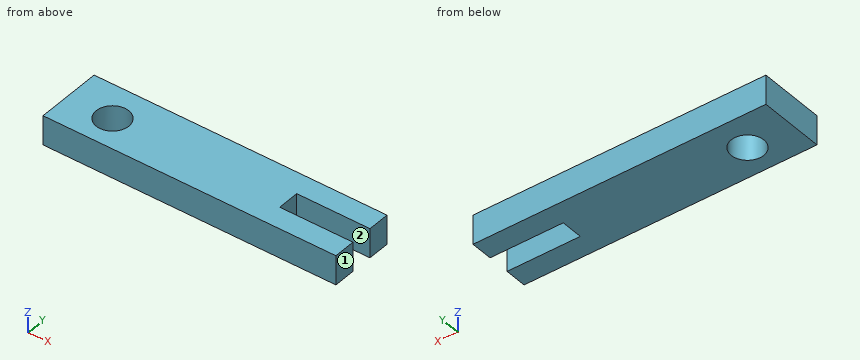
```python
from build123d import *

# Parameters (mm, degrees)
CROQUIS1_W              = 350
CROQUIS1_H              = 20
SALIENTE_EXTRUIR1_DEPTH = 45
CROQUIS2_R              = 11.125
CORTAR_EXTRUIR1_DEPTH   = 182.796589627
CROQUIS3_R              = 11.125
CORTAR_EXTRUIR2_DEPTH   = 182.796589627


with BuildPart() as part:
    # Croquis1 → Saliente-Extruir1 (new body)
    with BuildSketch(Plane(origin=(0, 0, 0), x_dir=(1, 0, 0), z_dir=(0, 1, 0))):
        Rectangle(CROQUIS1_W, CROQUIS1_H)
    extrude(amount=SALIENTE_EXTRUIR1_DEPTH)

    # Croquis2 → Cortar-Extruir1 (cut, through all)
    with BuildSketch(Plane(origin=(0, 0, -10), x_dir=(-1, 0, 0), z_dir=(0, 0, -1))):
        with Locations((-143.9, 21.1)):
            Circle(CROQUIS2_R)
    cortar_extruir1 = extrude(amount=-CORTAR_EXTRUIR1_DEPTH, mode=Mode.SUBTRACT)

    # Simetría1: Cortar-Extruir1 across plane
    add(cortar_extruir1.mirror(Plane(origin=(0, 0, 0), x_dir=(0, 0, 1), z_dir=(1, 0, 0))), mode=Mode.SUBTRACT)

    # Croquis3 → Cortar-Extruir2 (cut, through all)
    with BuildSketch(Plane.XY.offset(10)):
        Polygon((25, 15), (25, 0), (175, 0), (175, 45), (25, 45), (25, 30), (-25, 30), (-25, 15), align=None)
        with Locations((143.9, 21.1)):
            Circle(CROQUIS3_R, mode=Mode.SUBTRACT)
    extrude(amount=-CORTAR_EXTRUIR2_DEPTH, mode=Mode.SUBTRACT)


solid = part.part
```
The listing builds one solid part. Answer for the finished solid, in the listing's coordinates (mm). Face numbers are marked on the shaded views. A direction names the side the tool comes from. Coordinates: 2 decimals unless noted, no trailing zeros. Write each loop counter-clockwise with the first axis right and the second up, starting at its lowest first coordinate (ties: lowest second). Pieces come first, ordered by that corner, then holes.
Q1. Find the intervals of material crossed by line 1 along Y through (x, z) = (-23, 7); line 2 along X through (y, z) = (21.1, 0.5) (3 decimals); line 3 along Y through (x, z) = (-143.9, -4) (3 decimals), in increasing order.
Returned:
line 1: y = 0 to 15, 30 to 45
line 2: x = -175 to -155.025, -132.775 to -25
line 3: y = 0 to 9.975, 32.225 to 45
Q2. Section C-C, the plane z = 8.25 is taken. Write down the section's boundary in (x, y) (3 decimals), then the cut area to 3 significant figures.
Returned:
outline: (-175, 0) - (25, 0) - (25, 15) - (-25, 15) - (-25, 30) - (25, 30) - (25, 45) - (-175, 45) - close; hole circle Ø22.25 at (-143.9, 21.1)
area: 7,860 mm2
Q3. Section A-A, the plane x = -143.9 is taken. Write down the section's boundary in (y, z) (3 decimals), then the cut area to 3 significant figures.
Returned:
outline: (0, -10) - (9.975, -10) - (9.975, 10) - (0, 10) - close; (32.225, -10) - (45, -10) - (45, 10) - (32.225, 10) - close
area: 455 mm2
Q4. Section B-B, the plane y = 21.1 is taken. Write down the section's boundary in (x, z) (3 decimals).
Returned:
outline: (-175, -10) - (-155.025, -10) - (-155.025, 10) - (-175, 10) - close; (-132.775, -10) - (-25, -10) - (-25, 10) - (-132.775, 10) - close
Q5. Given P1, Ø2, axis at y = 23, z = 1, coming from the +X side, flat-ended and moving along its own axis, determine where the tip first touches the part or whether it passes through.
Returned:
P1: stops at x = -25
Q6. Which of the six approach directions +Z, -Z, +X, -X, +Y, -Y give full straight-line access (tool end or side, diameter ignored) to the marked faces 1 and 2?
Returned:
face 1: +Z, -Z, +X, +Y, -Y
face 2: +Z, -Z, +X
